from build123d import *

# Parameters (mm, degrees)
SKETCH1_R                  = 13.49375
BOSS_EXTRUDE1_DEPTH        = 6.35
F_10_32_TAPPED_HOLE1_D     = 4.0386
F_10_32_TAPPED_HOLE1_DEPTH = 12.02944
F_10_32_TAPPED_HOLE1_TIP   = 1.213317848


with BuildPart() as part:
    # Sketch1 → Boss-Extrude1 (new body, symmetric)
    with BuildSketch(Plane.XY):
        with BuildLine():
            Line((38.1, -44.45), (-38.1, -44.45))
            Line((-38.1, -44.45), (-38.1, 19.05))
            ThreePointArc((-38.1, 19.05), (-30.660512242, 37.010512242), (-12.7, 44.45))
            Line((-12.7, 44.45), (12.7, 44.45))
            ThreePointArc((12.7, 44.45), (30.660512242, 37.010512242), (38.1, 19.05))
            Line((38.1, 19.05), (38.1, -44.45))
        make_face()
        Circle(SKETCH1_R, mode=Mode.SUBTRACT)
    extrude(amount=BOSS_EXTRUDE1_DEPTH, both=True)

    # #10-32 Tapped Hole1
    with Locations(Plane(origin=(0, -44.45, 0), x_dir=(-1, 0, 0), z_dir=(0, -1, 0))):
        with Locations((19.05, 0), (-19.05, 0)):
            Hole(F_10_32_TAPPED_HOLE1_D / 2, depth=F_10_32_TAPPED_HOLE1_DEPTH)
            with Locations((0, 0, -(F_10_32_TAPPED_HOLE1_DEPTH + F_10_32_TAPPED_HOLE1_TIP / 2))):  # 118° drill point
                Cone(0, F_10_32_TAPPED_HOLE1_D / 2, F_10_32_TAPPED_HOLE1_TIP, mode=Mode.SUBTRACT)


solid = part.part
Work out the finished part from the listing and answer in its coordinate system (mm). A direction names the side the tool comes from. Coordinates: 2 decimals unless noted, no trailing zeros. Loops run counter-clockwise (first coordinate to the right, second up) from the corner with the lowest first, then second, coordinate; pieces in that order, holes last. Notation, with made-up numbers: (-28.75, -18) -> (-14.75, -18) arc R37 ccw to (-14.75, 20) -> close; hole circle Ø9 at (25.25, 38). An arc over 180 degrees is marked (long way). Write each question's results on one line, items separated by ' | '. Start each with the question number.
1) Find section A-A on x = 0. Determine the outline of the cut face in (y, z).
2) Consider line 1 along Z through (x, y) = (19, -36); line 2 along Y through (x, z) = (0, 1.5); line 3 along Y through (x, z) = (-5.5, 4). Determine where each line is inside the solid, lowest interval first.
3) Find section C-C on z = -3. Determine the outline of the cut face in (x, y).
4) Find section B-B on y = 0. Determine the outline of the cut face in (x, z).
5) Find section D-D on y = -35. Determine the outline of the cut face in (x, z).
6) Flat-ended cylindrical pins translate along their axes: P1, Ø4, axis at x = 19.5, z = 1.5, coming from the +Y side; P2, Ø5.5, axis at x = 19.05, z = 0, coming from the -Y side; P3, Ø5.5, axis at x = -19.05, z = 0, coming from the +Y side; P4, Ø1.5, axis at x = 29, z = -2.5, coming from the +Y side. Find the tip coordinate at first contact, or state that the pin passes through.
7) The mould has two halves that part along X. Classify faces 3 (the conical face through (18.716, -31.418, -0.105)), 4 (the flat face through (1, -44.45, 0)), 5 (the cylindrical face through (30.46, 37.21, 0.09)): pulls with the +X half, pulls with the -X half, needs draft (parallel to the pull), parting line crosses it, or undercut.
8) For faces 1 (the cylindrical face through (-17.124, -38.351, -0.607)), 2 (the flat face through (9, 11, -6.35)), determine the directions among +Z, -Z, +X, -X, +Y, -Y from which every point of the face is accessible in a straight line to the end or side of a thin tool.
Response values:
1) outline: (-44.45, -6.35) -> (-13.49, -6.35) -> (-13.49, 6.35) -> (-44.45, 6.35) -> close; (13.49, -6.35) -> (44.45, -6.35) -> (44.45, 6.35) -> (13.49, 6.35) -> close
2) line 1: z = -6.35 to -2.02, 2.02 to 6.35 | line 2: y = -44.45 to -13.49, 13.49 to 44.45 | line 3: y = -44.45 to -12.32, 12.32 to 44.45
3) outline: (-38.1, -44.45) -> (38.1, -44.45) -> (38.1, 19.05) arc R25.4 ccw to (12.7, 44.45) -> (-12.7, 44.45) arc R25.4 ccw to (-38.1, 19.05) -> close; hole circle Ø26.99 at (0, 0)
4) outline: (-38.1, -6.35) -> (-13.49, -6.35) -> (-13.49, 6.35) -> (-38.1, 6.35) -> close; (13.49, -6.35) -> (38.1, -6.35) -> (38.1, 6.35) -> (13.49, 6.35) -> close
5) outline: (-38.1, -6.35) -> (38.1, -6.35) -> (38.1, 6.35) -> (-38.1, 6.35) -> close; hole circle Ø4.04 at (-19.05, 0); hole circle Ø4.04 at (19.05, 0)
6) P1: stops at y = 43.99 | P2: stops at y = -44.45 | P3: stops at y = 44.19 | P4: stops at y = 39.13
7) face 3: undercut | face 4: needs draft | face 5: pulls with the +X half
8) face 1: -Y | face 2: -Z, +X, -X, +Y, -Y
